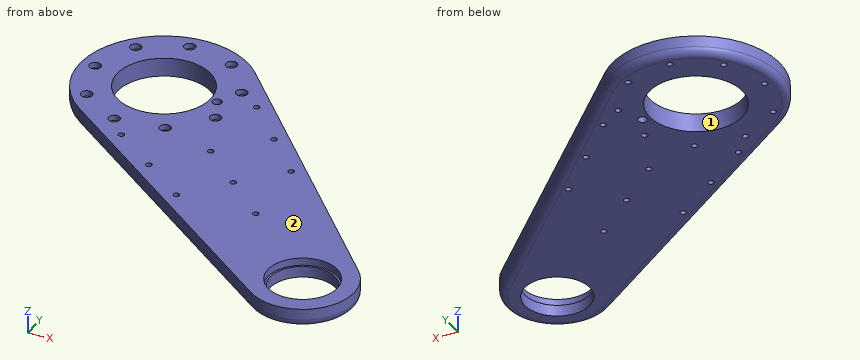
```python
from build123d import *

# Parameters (mm, degrees)
SKETCH1_R           = 17.5
SKETCH1_R_2         = 1.6
BOSS_EXTRUDE1_DEPTH = 10
SKETCH2_R           = 25
SKETCH2_R_2         = 2.5
SKETCH2_R_3         = 1.6
CUT_EXTRUDE1_DEPTH  = 224.991888552
SKETCH3_R           = 18.5625
CUT_EXTRUDE2_DEPTH  = 4
SKETCH4_R           = 3
CUT_EXTRUDE3_DEPTH  = 3
FILLET1_R           = 4


with BuildPart() as part:
    # Sketch1 → Boss-Extrude1 (new body)
    with BuildSketch(Plane.XY):
        with BuildLine():
            Line((-25.534872354, -37.053613776), (126.113577761, -141.559582877))
            ThreePointArc((126.113577761, -141.559582877), (162.784444163, -136.592367058), (161.308367688, -99.616065541))
            Line((161.308367688, -99.616065541), (32.056602073, 31.581232775))
            ThreePointArc((32.056602073, 31.581232775), (-34.47199994, 28.925442436), (-25.534872354, -37.053613776))
        make_face()
        with Locations((141.718221977, -118.915707792)):
            Circle(SKETCH1_R, mode=Mode.SUBTRACT)
        with Locations((70.859110989, -59.457853896)):
            Circle(SKETCH1_R_2, mode=Mode.SUBTRACT)
        with Locations((93.840444282, -78.741482187)):
            Circle(SKETCH1_R_2, mode=Mode.SUBTRACT)
        with Locations((47.877777695, -40.174225605)):
            Circle(SKETCH1_R_2, mode=Mode.SUBTRACT)
        with Locations((47.767990244, 4.946625931)):
            Circle(SKETCH1_R_2, mode=Mode.SUBTRACT)
        with Locations((3.423348889, -47.901259716)):
            Circle(SKETCH1_R_2, mode=Mode.SUBTRACT)
        with Locations((68.973861607, -16.273907044)):
            Circle(SKETCH1_R_2, mode=Mode.SUBTRACT)
        with Locations((90.17973297, -37.494440018)):
            Circle(SKETCH1_R_2, mode=Mode.SUBTRACT)
        with Locations((28.003855203, -65.100059364)):
            Circle(SKETCH1_R_2, mode=Mode.SUBTRACT)
        with Locations((52.584361518, -82.298859012)):
            Circle(SKETCH1_R_2, mode=Mode.SUBTRACT)
    extrude(amount=BOSS_EXTRUDE1_DEPTH)

    # Sketch2 → Cut-Extrude1 (cut, through all)
    with BuildSketch(Plane.XY.offset(10)):
        Circle(SKETCH2_R)
        with Locations((29, 0)):
            Circle(SKETCH2_R_2)
        with Locations((-37.5, 0)):
            Circle(SKETCH2_R_3)
        with Locations((-28.726666617, 24.104535363)):
            Circle(SKETCH2_R_3)
        with Locations((-6.511806663, 36.930290738)):
            Circle(SKETCH2_R_3)
        with Locations((18.75, 32.475952642)):
            Circle(SKETCH2_R_3)
        with Locations((35.238473279, 12.825755375)):
            Circle(SKETCH2_R_3)
        with Locations((35.238473279, -12.825755375)):
            Circle(SKETCH2_R_3)
        with Locations((18.75, -32.475952642)):
            Circle(SKETCH2_R_3)
        with Locations((-6.511806663, -36.930290738)):
            Circle(SKETCH2_R_3)
        with Locations((-28.726666617, -24.104535363)):
            Circle(SKETCH2_R_3)
    extrude(amount=-CUT_EXTRUDE1_DEPTH, mode=Mode.SUBTRACT)

    # Sketch3 → Cut-Extrude2 (cut)
    with BuildSketch(Plane.XY.offset(10)):
        with Locations((141.718221977, -118.915707792)):
            Circle(SKETCH3_R)
    extrude(amount=-CUT_EXTRUDE2_DEPTH, mode=Mode.SUBTRACT)

    # Sketch4 → Cut-Extrude3 (cut)
    with BuildSketch(Plane.XY.offset(10)):
        with Locations((-28.726666617, 24.104535363)):
            Circle(SKETCH4_R)
        with Locations((-6.511806663, 36.930290738)):
            Circle(SKETCH4_R)
        with Locations((18.75, 32.475952642)):
            Circle(SKETCH4_R)
        with Locations((35.238473279, 12.825755375)):
            Circle(SKETCH4_R)
        with Locations((35.238473279, -12.825755375)):
            Circle(SKETCH4_R)
        with Locations((18.75, -32.475952642)):
            Circle(SKETCH4_R)
        with Locations((-6.511806663, -36.930290738)):
            Circle(SKETCH4_R)
        with Locations((-28.726666617, -24.104535363)):
            Circle(SKETCH4_R)
        with Locations((-37.5, 0)):
            Circle(SKETCH4_R)
    extrude(amount=-CUT_EXTRUDE3_DEPTH, mode=Mode.SUBTRACT)

    # Fillet1
    fillet1_edges = [part.edges().sort_by_distance(p)[0] for p in [
        (96.68248488, -34.017416383, 0),
        (162.784444163, -136.592367058, 0),
        (50.289352703, -89.306598327, 0),
        (-34.47199994, 28.925442436, 0),
    ]]
    fillet(fillet1_edges, radius=FILLET1_R)


solid = part.part
```
Work out the finished part from the listing and answer in its coordinate system (mm). Face numbers are marked on the shaded views. Round coordinates to 2 decimals unless told otherwise and drop trailing zeros.
Q1. The mould has two halves that part along X. Classify the marked faces 1 and 2: pulls with the +X half, pulls with the -X half, needs draft (parallel to the pull), parting line crosses it, or undercut.
Solution:
face 1: undercut
face 2: needs draft
Q2. Find the intervals of material crossed by line 1 along X through (y, z) = (12.5, 4.25); line 2 along Y through (x, z) = (-30, 5.5); line 3 along Y through (x, z) = (-27.5, 5), in increasing order.
Solution:
line 1: x = -43.23 to -21.65, 21.65 to 33.67, 36.8 to 50.85
line 2: y = -33.54 to -25.07, -23.14 to 23.14, 25.07 to 33.54
line 3: y = -35.62 to -25.13, -23.08 to 23.08, 25.13 to 35.62
Q3. A cutting plane is placed at A-A, the plane z = 1.75. Count the separate pieces of the cut face and the enclosed holes in it, then the cut area to 3 significant figures.
Solution:
separate pieces: 1
enclosed holes: 21
area: 14,300 mm2
Q4. Given pin 1 Ø1 at (x, z) = (56, 4) entering from +Y; pin 2 Ø3 at (x, y) = (-7, -37) entering from +Z; pin 3 Ø4 at (x, z) = (103.5, 6) entering from +Y, each flat-ended and moving along its own axis, determine where each tip first touches the part or whether it passes through.
Solution:
pin 1: stops at y = 7.78
pin 2: stops at z = 7
pin 3: stops at y = -38.91
